from build123d import *

# Parameters (mm, degrees)
SKETCH_1_R      = 2.95
EXTRUDE_1_DEPTH = 9
SKETCH_2_R      = 1
EXTRUDE_2_DEPTH = 2
FILLET_1_R      = 2


with BuildPart() as part:
    # 草图1 → 凸台-拉伸1 (new body)
    with BuildSketch(Plane(origin=(0, 0, 0), x_dir=(1, 0, 0), z_dir=(0, 1, 0))):
        with Locations(Location((17.5, 0, 0), (0, 0, 270))):
            Circle(SKETCH_1_R)
    extrude(amount=EXTRUDE_1_DEPTH)

    # 草图2 → 凸台-拉伸2 (add)
    with BuildSketch(Plane(origin=(0, 0, 0), x_dir=(1, 0, 0), z_dir=(0, 1, 0))):
        Polygon((4.078263357, 14), (4.078263357, -14), (20, -14), (20.45, -14), (20.45, 14), (20, 14), align=None)
        with Locations(Location((10.5, -7, 0), (0, 0, 270))):
            Circle(SKETCH_2_R, mode=Mode.SUBTRACT)
        with Locations(Location((10.5, 7, 0), (0, 0, 270))):
            Circle(SKETCH_2_R, mode=Mode.SUBTRACT)
    extrude(amount=EXTRUDE_2_DEPTH)

    # 圆角1
    fillet_1_edges = [part.edges().sort_by_distance(p)[0] for p in [
        (4.078263357, 1, 14),
        (20.45, 1, 14),
        (20.45, 1, -14),
        (4.078263357, 1, -14),
    ]]
    fillet(fillet_1_edges, radius=FILLET_1_R)


solid = part.part
Model file for the job. Use its own axes, mm. A direction names the side the tool comes from. Coordinates: 2 decimals unless noted, no trailing zeros. Loops run counter-clockwise (first coordinate to the right, second up) from the corner with the lowest first, then second, coordinate; pieces in that order, holes last. Notation, with made-up numbers: (9, 28.25) -> (63, 28.25) arc R18 cw to (63, 40.25) -> close; hole circle Ø10 at (42.25, 64.25). An arc over 180 degrees is marked (long way). Use one line per item in the form item = value. Start each with the question number.
(1) Cut at C-C on x = 10.5. Give the cut face in (y, z).
(2) Cut at A-A on y = 1.25. Give the cut face in (x, z), and give its area (3 significant figures).
(3) Tool access for faces 4 (the cylindrical face through (4.65, 1.01, 13.4)), 5 (the cylindrical face through (19.987, 5.451, 1.586)): list every direction of +Z, -Z, +X, -X, +Y, -Y with a clear straight run to the whole face (end or side of a thin tool).
(4) Cut at D-D on x = 17.5. Give the cut face in (y, z), and give its area (3 significant figures).
(5) Pull direction X, two halves, no side cores. Call faces 1 (the cylindrical face through (11.49, 0.99, -7.13)), 2 (the flat face through (18, 9, 0)), 3 (the cylindrical face through (4.65, 1.01, -13.4)): pulls with the +X half, pulls with the -X half, needs draft (parallel to the pull), parting line crosses it, or undercut.
(6) Cut at B-B on z = -7. Give the cut face in (x, y), and give its area (3 significant figures).
(7) Probe probe 1 along X at (y, z) = (0.9, 7); probe 2 along Y at (x, z) = (13, 10); probe 3 along Z at (x, y) = (19.75, 3.25). List the from-to ranges inside material, lowest first. Write a range as from..to.
(8) Flat gauge pins, fed straight in: pin 1 (8 mm diameter, centred on x = 9, z = -2.5, fed in from +Y); pin 2 (2.5 mm diameter, centred on x = 10.5, z = -7, fed in from -Y); pin 3 (1.5 mm diameter, centred on x = 16.5, y = 3, fed in from +Z). Where does each tip first touch, or does it go through?
Values:
q1.outline = (0, -14) -> (2, -14) -> (2, -8) -> (0, -8) -> close; (0, -6) -> (2, -6) -> (2, 6) -> (0, 6) -> close; (0, 8) -> (2, 8) -> (2, 14) -> (0, 14) -> close
q2.outline = (4.08, -12) arc R2 ccw to (6.08, -14) -> (18.45, -14) arc R2 ccw to (20.45, -12) -> (20.45, 12) arc R2 ccw to (18.45, 14) -> (6.08, 14) arc R2 ccw to (4.08, 12) -> close; hole circle Ø2 at (10.5, -7); hole circle Ø2 at (10.5, 7)
q2.area = 449 mm2
q3.face_4 = +Z, -X, +Y, -Y
q3.face_5 = +Y
q4.outline = (0, -14) -> (2, -14) -> (2, -2.95) -> (9, -2.95) -> (9, 2.95) -> (2, 2.95) -> (2, 14) -> (0, 14) -> close
q4.area = 97.3 mm2
q5.face_1 = undercut
q5.face_2 = needs draft
q5.face_3 = pulls with the -X half
q6.outline = (4.08, 0) -> (9.5, 0) -> (9.5, 2) -> (4.08, 2) -> close; (11.5, 0) -> (20.45, 0) -> (20.45, 2) -> (11.5, 2) -> close
q6.area = 28.7 mm2
q7.probe_1 = 4.08..9.5, 11.5..20.45
q7.probe_2 = 0..2
q7.probe_3 = -1.91..1.91
q8.pin_1 = 2
q8.pin_2 = 0
q8.pin_3 = 2.94
